from build123d import *

# Parameters (mm, degrees)
CROQUIS1_R              = 1.65
CROQUIS1_R_2            = 14.9
SALIENTE_EXTRUIR1_DEPTH = 2.05


with BuildPart() as part:
    # Croquis1 → Saliente-Extruir1 (new body)
    with BuildSketch(Plane(origin=(0, 0, 0), x_dir=(0, 0, -1), z_dir=(1, 0, 0))):
        with BuildLine():
            Line((-15.25, -18.25), (15.25, -18.25))
            ThreePointArc((15.25, -18.25), (17.371320344, -17.371320344), (18.25, -15.25))
            Line((18.25, -15.25), (18.25, 15.25))
            ThreePointArc((18.25, 15.25), (17.371320344, 17.371320344), (15.25, 18.25))
            Line((15.25, 18.25), (-15.25, 18.25))
            ThreePointArc((-15.25, 18.25), (-17.371320344, 17.371320344), (-18.25, 15.25))
            Line((-18.25, 15.25), (-18.25, -15.25))
            ThreePointArc((-18.25, -15.25), (-17.371320344, -17.371320344), (-15.25, -18.25))
        make_face()
        with Locations((-15.1, 15.1)):
            Circle(CROQUIS1_R, mode=Mode.SUBTRACT)
        with Locations((-15.1, -15.1)):
            Circle(CROQUIS1_R, mode=Mode.SUBTRACT)
        with Locations((15.1, -15.1)):
            Circle(CROQUIS1_R, mode=Mode.SUBTRACT)
        with Locations((15.1, 15.1)):
            Circle(CROQUIS1_R, mode=Mode.SUBTRACT)
        Circle(CROQUIS1_R_2, mode=Mode.SUBTRACT)
    extrude(amount=SALIENTE_EXTRUIR1_DEPTH)

    # Croquis2 → Revolución1 (revolve)
    with BuildSketch(Plane.XY, mode=Mode.PRIVATE) as revoluci_n1_sk:
        Polygon((0, 14.9), (11.75, 14.9), (11.75, 12.875), (15.45, 12.875), (15.45, 13.575), (17.05, 13.575), (17.05, 11.685), (-3.25, 11.685), (-3.25, 9), (-8.7, 9), (-8.7, 13.6), (0, 13.6), align=None)
    revolve(revoluci_n1_sk.sketch.rotate(Axis((0, 0, 0), (1, 0, 0)), 90), axis=Axis((0, 0, 0), (1, 0, 0)))


solid = part.part
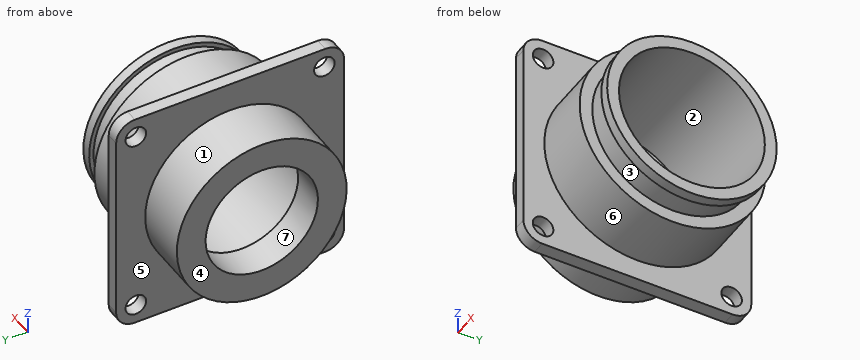
Geometry check sheet. Reference: the model listing, model coordinates, mm. Face numbers are marked on the shaded views. A direction names the side the tool comes from. Give positions to 0.01 mm unless a question says otherwise; leave off trailing zeros. Write each loop counter-clockwise with the first axis right and the second up, starting at its lowest first coordinate (ties: lowest second). Pieces come first, ordered by that corner, then holes.
1) Release check for a two-part mould opening along Z. For the marked faces 5, 6 and 7 record: released by +Z, released by -Z, zero draft, split by the parting line, or undercut.
Values follow:
face 5: zero draft
face 6: split by the parting line
face 7: undercut
2) Thickness scan on line 1 (X direction, y = -8.5, z = 10.5); line 2 (Y direction, x = 1.15, z = -15.1); line 3 (Y direction, x = 0.5, z = -14). Record the ranges inside material, lowest first.
Values follow:
line 1: x = -8.7 to 11.75, 15.45 to 17.05
line 2: y = -18.25 to -16.75, -13.45 to 13.45, 16.75 to 18.25
line 3: y = -18.25 to -16.33, -13.87 to 13.87, 16.33 to 18.25
3) Set-up check for the marked faces 1, 2, 3 and 4: record each of +Z, -Z, +X, -X, +Y, -Y from which the full face is reachable in a straight line by a thin tool's end or side.
Values follow:
face 1: -X
face 2: +X
face 3: none
face 4: +Z, -Z, -X, +Y, -Y
4) Cross-section at C-C (x = 7.75). Record the boundary of the cut face in (y, z) (3 decimals), plus the area to 3 significant figures.
Values follow:
outline: circle Ø29.8 at (0, 0); hole circle Ø23.37 at (0, 0)
area: 269 mm2
5) Cross-section at A-A (y = 0). Record the boundary of the cut face in (x, z) (3 decimals), plus the area to 3 significant figures.
Values follow:
outline: (-8.7, -13.6) - (0, -13.6) - (0, -18.25) - (2.05, -18.25) - (2.05, -14.9) - (11.75, -14.9) - (11.75, -12.875) - (15.45, -12.875) - (15.45, -13.575) - (17.05, -13.575) - (17.05, -11.685) - (-3.25, -11.685) - (-3.25, -9) - (-8.7, -9) - close; (-8.7, 9) - (-3.25, 9) - (-3.25, 11.685) - (17.05, 11.685) - (17.05, 13.575) - (15.45, 13.575) - (15.45, 12.875) - (11.75, 12.875) - (11.75, 14.9) - (2.05, 14.9) - (2.05, 18.25) - (0, 18.25) - (0, 13.6) - (-8.7, 13.6) - close
area: 167 mm2
6) Go/stop test with flat-tipped pins: pin 1 Ø5.5 at (y, z) = (15.1, -15.1) entering from +X; pin 2 Ø8 at (x, y) = (-5, -4) entering from +Z; pin 3 Ø6 at (x, z) = (10, -3) entering from +Y. Record where each tip stops, or that it passes through.
Values follow:
pin 1: stops at x = 2.05
pin 2: stops at z = 13.6
pin 3: stops at y = 14.9
7) Cross-section at D-D (z = 11). Record the boundary of the cut face in (x, y), plus the area to 3 significant figures.
Values follow:
outline: (-8.7, -8) - (0, -8) - (0, -18.25) - (2.05, -18.25) - (2.05, -10.05) - (11.75, -10.05) - (11.75, -6.69) - (15.45, -6.69) - (15.45, -7.95) - (17.05, -7.95) - (17.05, -3.94) - (-3.25, -3.94) - (-3.25, 3.94) - (17.05, 3.94) - (17.05, 7.95) - (15.45, 7.95) - (15.45, 6.69) - (11.75, 6.69) - (11.75, 10.05) - (2.05, 10.05) - (2.05, 18.25) - (0, 18.25) - (0, 8) - (-8.7, 8) - close
area: 324 mm2
